Check sheet for the modelled part. Datum: model origin and axes. Units: mm. Coordinates: 2 decimals unless noted, no trailing zeros. Order: outer loops, then holes, each group sorted by start corner. A loop starts at its lowest first (then second) coordinate and runs counter-clockwise, first axis right, second up.
from build123d import *

# Parameters (mm, degrees)
F0_R     = 17.1
F0_R_2   = 16.5
F1_DEPTH = 5.5
F2_DEPTH = 0.5
F3_R     = 1


with BuildPart() as f1:
    # F0 (on Front) → F1 (new body)
    with BuildSketch(Plane.XZ):
        Circle(F0_R)
        Circle(F0_R_2, mode=Mode.SUBTRACT)
    extrude(amount=F1_DEPTH)

    # F0 (on Front) → F2 (join)
    with BuildSketch(Plane.XZ):
        Circle(F0_R_2)
    extrude(amount=F2_DEPTH)

    # F3
    f3_edges = [f1.edges().sort_by_distance(p)[0] for p in [
        (-17.1, 0, 0),
    ]]
    fillet(f3_edges, radius=F3_R)


solid = f1.part
(1) Release check for a two-part mould opening along X. For faces 1 (the flat face through (0, -0.5, 0)), 2 (the flat face through (0, 0, 0)), 3 (the cylindrical face through (16.31, -3.22, 5.14)) record: +X half, -X half, draft (parallel to the pull), parting line (faces both ways), or undercut.
Filled in:
face 1: undercut
face 2: draft
face 3: parting line
(2) Cross-section at A-A (x = 0). Enter the section's corners in (y, z).
Filled in:
outline: (-5.5, -17.1) - (-1, -17.1) arc R1 ccw to (0, -16.1) - (0, 16.1) arc R1 ccw to (-1, 17.1) - (-5.5, 17.1) - (-5.5, 16.5) - (-0.5, 16.5) - (-0.5, -16.5) - (-5.5, -16.5) - close
(3) Cross-section at C-C (z = 0). Enter the section's corners in (x, y).
Filled in:
outline: (-17.1, -5.5) - (-16.5, -5.5) - (-16.5, -0.5) - (16.5, -0.5) - (16.5, -5.5) - (17.1, -5.5) - (17.1, -1) arc R1 ccw to (16.1, 0) - (-16.1, 0) arc R1 ccw to (-17.1, -1) - close
(4) Cross-section at B-B (y = -1.55). Enter the section's corners in (x, z).
Filled in:
outline: circle Ø34.2 at (0, 0); hole circle Ø33 at (0, 0)
(5) Go/stop test with flat-tipped pins: P1, Ø1, axis at x = -12, y = -3.5, coming from the -Z side; P2, Ø1, axis at x = 13, z = -5, coming from the -Y side. Record where each tip stops, or that it passes through.
Filled in:
P1: stops at z = -12.66
P2: stops at y = -0.5
(6) Thickness scan on probe 1 along Z at (x, y) = (0, -2.45); probe 2 along Y at (x, z) = (12, 4.5); probe 3 along Z at (x, y) = (4, -2.1). Record the ranges inside material, lowest first.
Filled in:
probe 1: z = -17.1 to -16.5, 16.5 to 17.1
probe 2: y = -0.5 to 0
probe 3: z = -16.63 to -16.01, 16.01 to 16.63
